from build123d import *

# Parameters (mm, degrees)
CROQUIS1_R              = 1.8
SALIENTE_EXTRUIR1_DEPTH = 1


with BuildPart() as part:
    # Croquis1 → Saliente-Extruir1 (new body)
    with BuildSketch(Plane.XY):
        with BuildLine():
            ThreePointArc((-26.248809497, 20), (-33, 0), (-26.248809497, -20))
            Line((-26.248809497, -20), (17, -20))
            Line((17, -20), (17, 20))
            Line((17, 20), (-26.248809497, 20))
        make_face()
        with Locations((-29, 0)):
            Circle(CROQUIS1_R, mode=Mode.SUBTRACT)
    extrude(amount=SALIENTE_EXTRUIR1_DEPTH)


solid = part.part
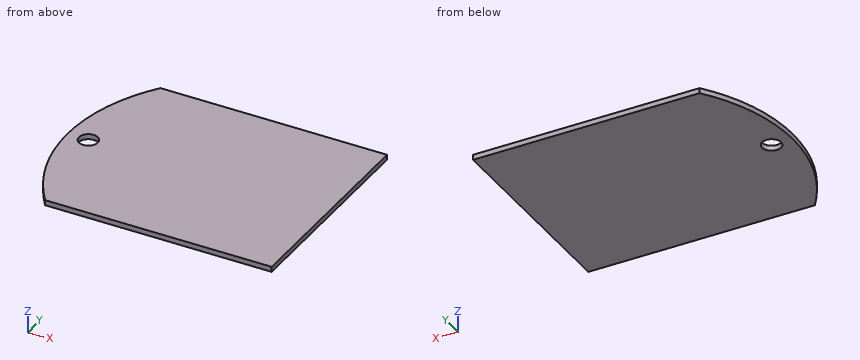
The listing builds one solid part. Answer for the finished solid, in the listing's coordinates (mm). Round coordinates to 2 decimals unless told otherwise and drop trailing zeros. Write each loop counter-clockwise with the first axis right and the second up, starting at its lowest first coordinate (ties: lowest second). Pieces come first, ordered by that corner, then holes. Notation, with made-up numbers: (-21, 65) - (-14, 65) arc R10 cw to (-14, 82) - close; hole circle Ø3 at (23, -38.5). An arc over 180 degrees is marked (long way). Use a Markdown table: item, result. Add a question column.
1. Consider line 1 (Y direction, x = -29, z = 0.55); line 2 (X direction, y = -1, z = 0.8); line 3 (Y direction, x = -27.5, z = 0.3). Determine where each line is inside the solid, lowest interval first.
2. The part is cut by section D-D (y = -9.5). Write down the section's boundary in (x, z).
3. The part is cut by section C-C (z = 0.2). Write down the section's boundary in (x, y), and give its area (3 significant figures).
4. The part is cut by section A-A (y = 0). Write down the section's boundary in (x, z), and give its area (3 significant figures).
5. The part is cut by section B-B (x = -29). Write down the section's boundary in (y, z).
Reported:
| question | item | result |
|---|---|---|
| 1 | line 1 | -15.75 to -1.8, 1.8 to 15.75 |
| 1 | line 2 | -32.98 to -30.5, -27.5 to 17 |
| 1 | line 3 | -18.24 to -0.99, 0.99 to 18.24 |
| 2 | outline | (-31.6, 0) - (17, 0) - (17, 1) - (-31.6, 1) - close |
| 3 | outline | (-26.25, -20) - (17, -20) - (17, 20) - (-26.25, 20) arc R33 ccw to start; hole circle Ø3.6 at (-29, 0) |
| 3 | area | 1,900 mm^2 |
| 4 | outline | (-33, 0) - (-30.8, 0) - (-30.8, 1) - (-33, 1) - close; (-27.2, 0) - (17, 0) - (17, 1) - (-27.2, 1) - close |
| 4 | area | 46.4 mm^2 |
| 5 | outline | (-15.75, 0) - (-1.8, 0) - (-1.8, 1) - (-15.75, 1) - close; (1.8, 0) - (15.75, 0) - (15.75, 1) - (1.8, 1) - close |
